Answer from the drawing. Dimensions are ordinates in mm from the lowest x, y and z of the part. A direction names the side the tool comes from. Coordinates: 2 decimals unless noted, no trailing zeros. Loops run counter-clockwise (first coordinate to the right, second up) from the corner with the lowest first, then second, coordinate; pieces in that order, holes last. Notation, with made-up numbers: (41.25, 76) - (57.25, 76) arc R18 cw to (57.25, 90) - close; hole circle Ø5 at (8, -35.5). An arc over 180 degrees is marked (long way). Write each question's results on one line, items separated by ' | '. Start each with the question number.
1. Find the intervals of material crossed by line 1 along X through (y, z) = (6.25, 23); line 2 along Z through (x, y) = (20.5, 0.5); line 3 along Z through (x, y) = (23, 3), in increasing order. Write a range as [from, to].
2. A cutting plane is placed at A-A on x = 23. Determine the outline of the cut face in (y, z).
3. A cutting plane is placed at B-B on z = 23. Determine the outline of the cut face in (x, y).
4. Determine the mould class of the marked faces 3, 4 and 5 for opening direction Z: released by +Z, released by -Z, zero draft, split by the parting line, or undercut.
5. A cutting plane is placed at D-D on y = 2. Determine the outline of the cut face in (x, z), then the cut area to 3 significant figures.
6. Each of these flat-tipped pins is pushed along its axis until it touches: P1, Ø4, axis at y = 6.5, z = 15, coming from the +X side; P2, Ø6, axis at x = 5.5, z = 23, coming from the -Y side; P3, Ø4.5, axis at x = 23, z = 40.5, coming from the +Y side; P4, Ø6.5, axis at x = 40.5, z = 23, coming from the +Y side. Where does it stop, or does it pass through?
7. A cutting plane is placed at C-C on z = 5.5. Determine the outline of the cut face in (x, y).
8. Which of the six approach directions +Z, -Z, +X, -X, +Y, -Y give full straight-line access (tool end or side, diameter ignored) to the marked faces 1 and 2?
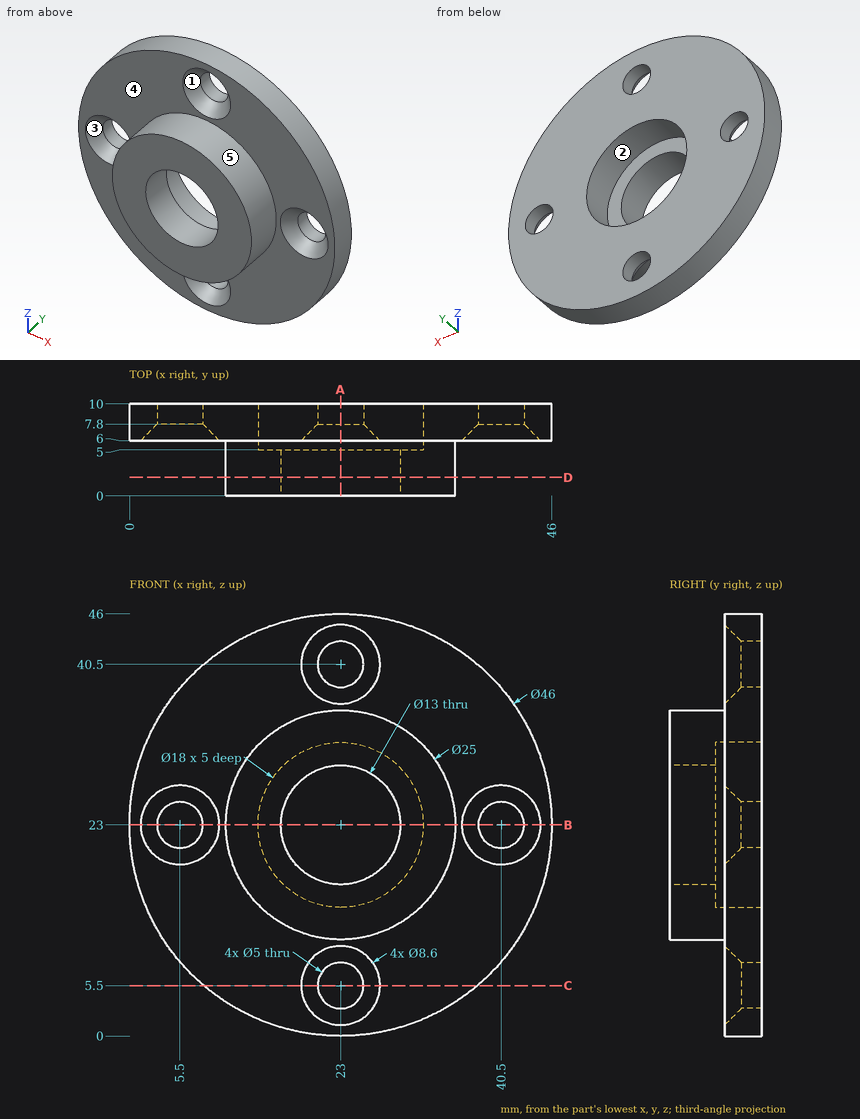
Values:
1) line 1: [0, 1.45], [9.55, 14], [32, 36.45], [44.55, 46] | line 2: [10.75, 17], [29, 35.25] | line 3: [10.5, 16.5], [29.5, 35.5]
2) outline: (0, 10.5) - (6, 10.5) - (6, 9.8) - (7.8, 8) - (10, 8) - (10, 14) - (5, 14) - (5, 16.5) - (0, 16.5) - close; (0, 29.5) - (5, 29.5) - (5, 32) - (10, 32) - (10, 38) - (7.8, 38) - (6, 36.2) - (6, 35.5) - (0, 35.5) - close; (6, 0) - (10, 0) - (10, 3) - (7.8, 3) - (6, 1.2) - close; (6, 44.8) - (7.8, 43) - (10, 43) - (10, 46) - (6, 46) - close
3) outline: (0, 6) - (1.2, 6) - (3, 7.8) - (3, 10) - (0, 10) - close; (8, 7.8) - (9.8, 6) - (10.5, 6) - (10.5, 0) - (16.5, 0) - (16.5, 5) - (14, 5) - (14, 10) - (8, 10) - close; (29.5, 0) - (35.5, 0) - (35.5, 6) - (36.2, 6) - (38, 7.8) - (38, 10) - (32, 10) - (32, 5) - (29.5, 5) - close; (43, 7.8) - (44.8, 6) - (46, 6) - (46, 10) - (43, 10) - close
4) face 3: undercut | face 4: zero draft | face 5: split by the parting line
5) outline: circle Ø25 at (23, 23); hole circle Ø13 at (23, 23) | area: 358 mm^2
6) P1: x = 45.2 | P2: y = 7.3 | P3: through | P4: y = 10
7) outline: (8.08, 6) - (18.7, 6) - (20.5, 7.8) - (20.5, 10) - (8.08, 10) - close; (25.5, 7.8) - (27.3, 6) - (37.92, 6) - (37.92, 10) - (25.5, 10) - close
8) face 1: -Y | face 2: +Y
